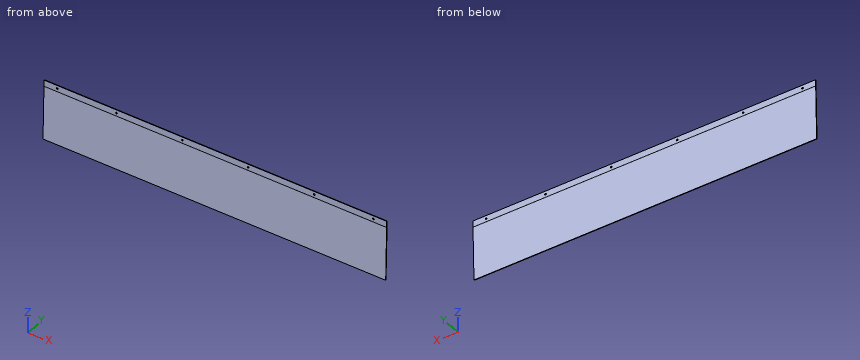
from build123d import *

# Parameters (mm, degrees)
F1_DEPTH    = 650
F2_R        = 3.25
F3_DEPTH    = 25
F4_T1_DEPTH = 1300
F5_T1_DEPTH = 1300.2618143417


# Not quite as in the source:
# - a fillet or chamfer that OpenCascade refuses, or shapes differently, is made with other operations: its cross-section is extruded or revolved along the edge and cut away or added


with BuildPart() as f1:
    # F0 (on Right) → F1 (new body, symmetric)
    with BuildSketch(Plane.YZ):
        Polygon((0, -24), (0, 0), (-2, 0), (-2, -23.9738185658), (-7.2608812598, -224.8787684235), (-5.2615666099, -224.9311223201), align=None)
    extrude(amount=F1_DEPTH, both=True)

    # F2 (on face) → F3 (cut)
    with BuildSketch(Plane(origin=(0, 0, 0), x_dir=(-1, 0, 0), z_dir=(0, 1, 0))):
        with Locations((-600, -12)):
            Circle(F2_R)
        with Locations((-375, -12)):
            Circle(F2_R)
        with Locations((-125, -12)):
            Circle(F2_R)
        with Locations((600, -12)):
            Circle(F2_R)
        with Locations((375, -12)):
            Circle(F2_R)
        with Locations((125, -12)):
            Circle(F2_R)
    extrude(amount=-F3_DEPTH, mode=Mode.SUBTRACT)

    # F4: fillet of radius 2 on 1 edges, made by hand

    # F4_s2 → F4_t1 (join)
    with BuildSketch(Plane.YZ.offset(-650)):
        with BuildLine():
            ThreePointArc((-2, -23.9476371317), (-2.0001713449, -23.9738163228), (-2.00068535, -23.9999910283))
            Line((-2.00068535, -23.9999910283), (-2, -23.9738185658))
            Line((-2, -23.9738185658), (-2, -23.9476371317))
        make_face()
    extrude(amount=F4_T1_DEPTH)

    # F5: fillet of radius 4 on 1 edges, made by hand

    # F5_s2 → F5_t1 (cut)
    with BuildSketch(Plane.YZ.offset(-650.1309071708)):
        with BuildLine():
            ThreePointArc((-0.0013707001, -24.0523449249), (-0.0003426897, -23.9999955139), (0, -23.9476371317))
            Line((0, -23.9476371317), (0, -24))
            Line((0, -24), (-0.0013707001, -24.0523449249))
        make_face()
    extrude(amount=F5_T1_DEPTH, mode=Mode.SUBTRACT)


solid = f1.part
The listing builds one solid part. Answer for the finished solid, in the listing's coordinates (mm). Coordinates: 2 decimals unless noted, no trailing zeros. Loops run counter-clockwise (first coordinate to the right, second up) from the corner with the lowest first, then second, coordinate; pieces in that order, holes last. Notation, with made-up numbers: (15.25, 61.25) -> (47.25, 61.25) arc R31 ccw to (47.25, 85.25) -> close; hole circle Ø9 at (60, 37). An arc over 180 degrees is marked (long way). Answer in a Markdown table with one row per item. Add a question column.
1. The part is cut by section A-A, the plane x = -501. Write down the section's boundary in (y, z).
2. Consider line 1 (Y direction, x = 536.5, z = -32); line 2 (Y direction, x = 44, z = -103). Determine where each line is inside the solid, lowest interval first. Write a range as [from, to].
3. The part is cut by section B-B, the plane z = -109. Write down the section's boundary in (x, y), then the cut area to 3 significant figures.
4. Flat-ended cylindrical pins translate along their axes: P1, Ø6, axis at x = -125, z = -12, coming from the -Y side; P2, Ø3, axis at x = 206.5, z = -149.5, coming from the +Y side; P3, Ø6, axis at x = -171, z = -191.5, coming from the +Y side; P4, Ø5, axis at x = 71, z = -71, coming from the -Y side. Find the tip coordinate at first contact, or state that the pin passes through.
Answer below:
| question | item | result |
|---|---|---|
| 1 | outline | (-7.26, -224.88) -> (-5.26, -224.93) -> (0, -24.05) arc R4 ccw to (0, -23.95) -> (0, 0) -> (-2, 0) -> (-2, -23.95) arc R2 cw to (-2, -24) -> close |
| 2 | line 1 | [-2.21, -0.21] |
| 2 | line 2 | [-4.07, -2.07] |
| 3 | outline | (-650, -4.23) -> (650, -4.23) -> (650, -2.23) -> (-650, -2.23) -> close |
| 3 | area | 2,600 mm2 |
| 4 | P1 | through |
| 4 | P2 | y = -3.25 |
| 4 | P3 | y = -4.31 |
| 4 | P4 | y = -3.3 |
